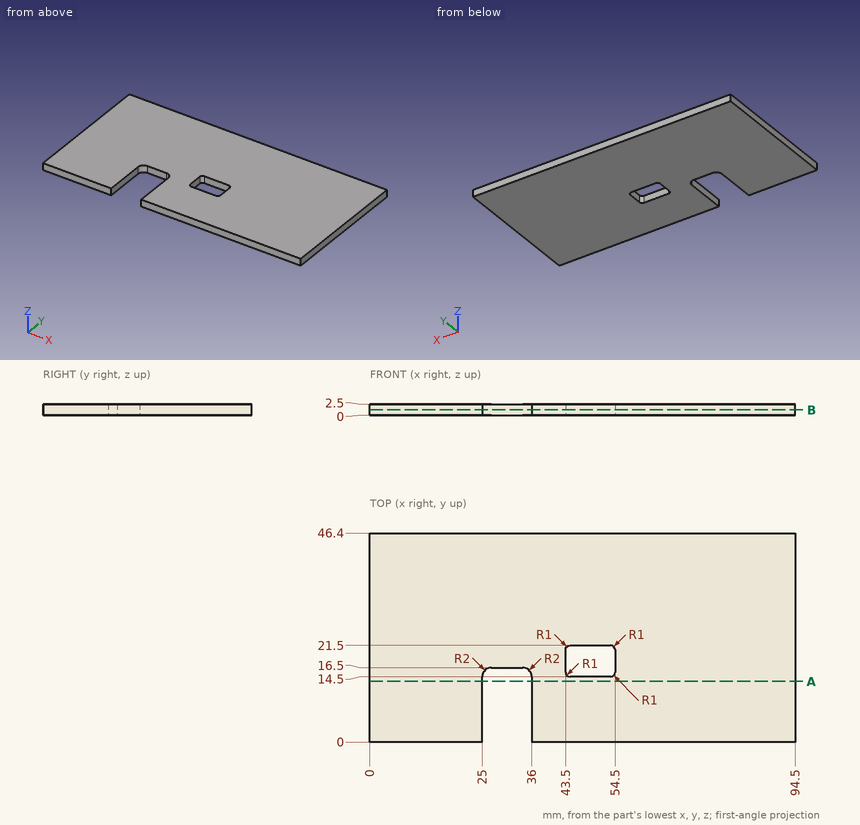
Answer from the drawing. Dimensions are ordinates in mm from the lowest x, y and z of the part. Coordinates: 2 decimals unless noted, no trailing zeros. Loops run counter-clockwise (first coordinate to the right, second up) from the corner with the lowest first, then second, coordinate; pieces in that order, holes last. Notation, with made-up numbers: (41, 24.5) -> (57, 24.5) arc R18 ccw to (57, 40.5) -> close; hole circle Ø3 at (78.5, 59.5). An arc over 180 degrees is marked (long way). Return JSON: item names as keys, results as strings.
Item 1: A flat-ended cylindrical pin translates along its axis: P1, Ø1.2, axis at x = 32, z = 1.5, coming from the -Y side. Find the tip coordinate at first contact, or state that the pin passes through.
Answers:
{"P1": "stops at y = 16.5"}
Item 2: Find section B-B (z = 1.2). Determine the outline of the cut face in (x, y).
Answers:
{"outline": "(0, 0) -> (25, 0) -> (25, 14.5) arc R2 cw to (27, 16.5) -> (34, 16.5) arc R2 cw to (36, 14.5) -> (36, 0) -> (94.5, 0) -> (94.5, 46.4) -> (0, 46.4) -> close; hole (43.5, 15.5) arc R1 ccw to (44.5, 14.5) -> (53.5, 14.5) arc R1 ccw to (54.5, 15.5) -> (54.5, 20.5) arc R1 ccw to (53.5, 21.5) -> (44.5, 21.5) arc R1 ccw to (43.5, 20.5) -> close"}
Item 3: Find section A-A (y = 13.5). Determine the outline of the cut face in (x, z).
Answers:
{"outline": "(0, 0) -> (25, 0) -> (25, 2.5) -> (0, 2.5) -> close; (36, 0) -> (94.5, 0) -> (94.5, 2.5) -> (36, 2.5) -> close"}
Item 4: Find the intervals of material crossed by probe 1 along X at (y, z) = (3, 0.25); probe 2 along Y at (x, z) = (45, 2.1); probe 3 along Y at (x, z) = (30.5, 0.6), in increasing order.
Answers:
{"probe 1": "x = 0 to 25, 36 to 94.5", "probe 2": "y = 0 to 14.5, 21.5 to 46.4", "probe 3": "y = 16.5 to 46.4"}
